Job drawing, mm, ordinate dimensions from the low corner. One solid piece. A direction names the side the tool comes from. Round coordinates to 2 decimals unless told otherwise and drop trailing zeros. Write each loop counter-clockwise with the first axis right and the second up, starting at its lowest first coordinate (ties: lowest second). Pieces come first, ordered by that corner, then holes. Notation, with made-up numbers: (-16.5, 20) - (42.5, 20) arc R6 cw to (42.5, 27) - close; hole circle Ø5 at (-25, 40). An arc over 180 degrees is marked (long way). Write each question's results on one line, items separated by ' | '.
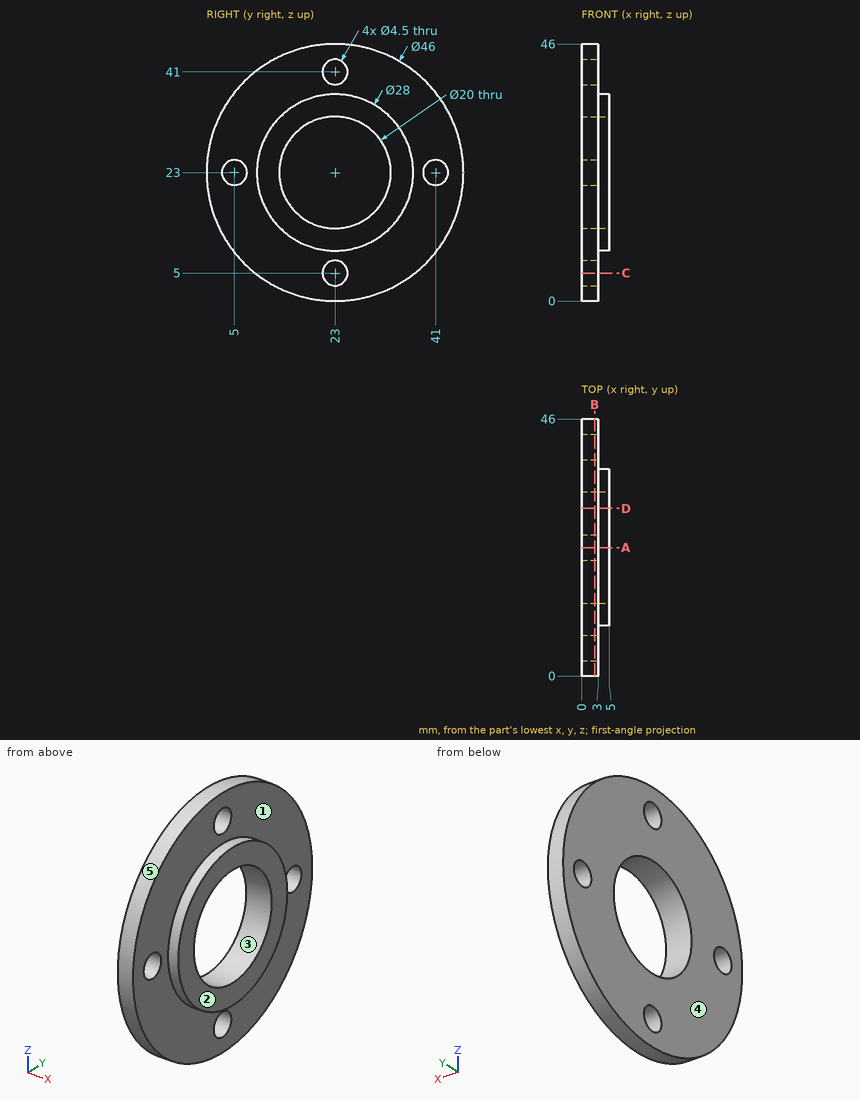
(1) Slice it at D-D, the plane y = 30. Write the cut outline in (x, z), and give its area (3 significant figures).
Worked answers:
outline: (0, 1.09) - (3, 1.09) - (3, 10.88) - (5, 10.88) - (5, 15.86) - (0, 15.86) - close; (0, 30.14) - (5, 30.14) - (5, 35.12) - (3, 35.12) - (3, 44.91) - (0, 44.91) - close | area: 109 mm2
(2) Two-plate mould, pull along Z, no slides. Class the marked faces 3, 4 and 5: released by +Z, released by -Z, zero draft, split by the parting line, or undercut.
Worked answers:
face 3: undercut | face 4: zero draft | face 5: split by the parting line
(3) Flat gauge pin, fed straight in: pin 1 Ø4 at (y, z) = (23, 41) entering from +X. Where does the tip first touch, or does it go through?
Worked answers:
pin 1: passes through
(4) Slice it at C-C, the plane z = 5. Write the cut outline in (x, y).
Worked answers:
outline: (0, 8.68) - (3, 8.68) - (3, 20.75) - (0, 20.75) - close; (0, 25.25) - (3, 25.25) - (3, 37.32) - (0, 37.32) - close
(5) Drill centre lines: probe 1 along Z at (x, y) = (2.2, 23); probe 2 along Z at (x, y) = (3.3, 23); probe 3 along X at (y, z) = (27.5, 5). Where is each one in solid material? Low to high. Write a range as [from, to].
Worked answers:
probe 1: z = [0, 2.75], [7.25, 13], [33, 38.75], [43.25, 46] | probe 2: z = [9, 13], [33, 37] | probe 3: x = [0, 3]
(6) Slice it at A-A, the plane y = 23. Write the cut outline in (x, z), and give its area (3 significant figures).
Worked answers:
outline: (0, 0) - (3, 0) - (3, 2.75) - (0, 2.75) - close; (0, 7.25) - (3, 7.25) - (3, 9) - (5, 9) - (5, 13) - (0, 13) - close; (0, 33) - (5, 33) - (5, 37) - (3, 37) - (3, 38.75) - (0, 38.75) - close; (0, 43.25) - (3, 43.25) - (3, 46) - (0, 46) - close | area: 67.0 mm2
(7) Slice it at B-B, the plane x = 2.35. Write the cut outline in (y, z).
Worked answers:
outline: circle Ø46 at (23, 23); hole circle Ø4.5 at (5, 23); hole circle Ø20 at (23, 23); hole circle Ø4.5 at (23, 5); hole circle Ø4.5 at (23, 41); hole circle Ø4.5 at (41, 23)
(8) Tool access for the marked faces 1 and 2: list every direction of +Z, -Z, +X, -X, +Y, -Y with a clear straight run to the whole face (end or side of a thin tool).
Worked answers:
face 1: +X | face 2: +Z, -Z, +X, +Y, -Y
